from build123d import *

# Parameters (mm, degrees)
SKETCH1_R               = 101.6
BOSS_EXTRUDE1_DEPTH     = 76.2
FILLET1_R               = 12.7
CUT_EXTRUDE1_DEPTH      = 163.639355693
CUT_EXTRUDE1_DEPTH_BACK = 163.639355693
CUT_EXTRUDE2_DEPTH      = 163.63935574
CUT_EXTRUDE2_DEPTH_BACK = 163.63935574
SKETCH5_R               = 12.7


with BuildPart() as part:
    # Sketch1 → Boss-Extrude1 (new body)
    with BuildSketch(Plane.YZ):
        with Locations(Location((0, 0, 0), (0, 0, 90))):
            Circle(SKETCH1_R)
    extrude(amount=BOSS_EXTRUDE1_DEPTH)

    # Fillet1
    fillet1_edges = [part.edges().sort_by_distance(p)[0] for p in [
        (0, 0, -101.6),
        (76.2, 0, -101.6),
    ]]
    fillet(fillet1_edges, radius=FILLET1_R)

    # Sketch2 → Cut-Extrude1 (cut, two sides: drawn at the far end of the back side and taken through both)
    with BuildSketch(Plane.YZ.offset(76.2).offset(-CUT_EXTRUDE1_DEPTH_BACK)):
        with BuildLine():
            ThreePointArc((-24.232427185, 7.612455104), (-25.4, 0), (-24.232427185, -7.612455104))
            add(Edge.make_bspline(
                [(-24.232427185, -7.612455104), (-44.761154303, -23.370868648), (-69.597655338, -31.025898399)],
                knots=[0, 0, 0, 1, 1, 1], degree=2))
            ThreePointArc((-69.597655338, -31.025898399), (-76.2, 0), (-69.597655338, 31.025898399))
            add(Edge.make_bspline(
                [(-24.232427185, 7.612455104), (-44.761154303, 23.370868648), (-69.597655338, 31.025898399)],
                knots=[0, 0, 0, 1, 1, 1], degree=2))
        make_face()
        with BuildLine():
            ThreePointArc((18.708793098, 17.179669986), (12.7, 21.997045256), (5.523634087, 24.79212509))
            add(Edge.make_bspline(
                [(5.523634087, 24.79212509), (2.140811193, 50.449731053), (7.92961148, 75.786286766)],
                knots=[0, 0, 0, 1, 1, 1], degree=2))
            ThreePointArc((7.92961148, 75.786286766), (38.1, 65.991135768), (61.668043858, 44.760388367))
            add(Edge.make_bspline(
                [(18.708793098, 17.179669986), (42.620343109, 27.078862405), (61.668043858, 44.760388367)],
                knots=[0, 0, 0, 1, 1, 1], degree=2))
        make_face()
        with BuildLine():
            ThreePointArc((24.232427185, -7.612455104), (25.4, 0), (24.232427185, 7.612455104))
            add(Edge.make_bspline(
                [(24.232427185, 7.612455104), (44.761154303, 23.370868648), (69.597655338, 31.025898399)],
                knots=[0, 0, 0, 1, 1, 1], degree=2))
            ThreePointArc((69.597655338, 31.025898399), (76.2, 0), (69.597655338, -31.025898399))
            add(Edge.make_bspline(
                [(24.232427185, -7.612455104), (44.761154303, -23.370868648), (69.597655338, -31.025898399)],
                knots=[0, 0, 0, 1, 1, 1], degree=2))
        make_face()
        with BuildLine():
            ThreePointArc((-61.668043858, -44.760388367), (-38.1, -65.991135768), (-7.92961148, -75.786286766))
            add(Edge.make_bspline(
                [(-5.523634087, -24.79212509), (-2.140811193, -50.449731053), (-7.92961148, -75.786286766)],
                knots=[0, 0, 0, 1, 1, 1], degree=2))
            ThreePointArc((-5.523634087, -24.79212509), (-12.7, -21.997045256), (-18.708793098, -17.179669986))
            add(Edge.make_bspline(
                [(-18.708793098, -17.179669986), (-42.620343109, -27.078862405), (-61.668043858, -44.760388367)],
                knots=[0, 0, 0, 1, 1, 1], degree=2))
        make_face()
        with BuildLine():
            ThreePointArc((5.523634087, -24.79212509), (12.7, -21.997045256), (18.708793098, -17.179669986))
            add(Edge.make_bspline(
                [(18.708793098, -17.179669986), (42.620343109, -27.078862405), (61.668043858, -44.760388367)],
                knots=[0, 0, 0, 1, 1, 1], degree=2))
            ThreePointArc((61.668043858, -44.760388367), (38.1, -65.991135768), (7.92961148, -75.786286766))
            add(Edge.make_bspline(
                [(5.523634087, -24.79212509), (2.140811193, -50.449731053), (7.92961148, -75.786286766)],
                knots=[0, 0, 0, 1, 1, 1], degree=2))
        make_face()
        with BuildLine():
            ThreePointArc((-7.92961148, 75.786286766), (-38.1, 65.991135768), (-61.668043858, 44.760388367))
            add(Edge.make_bspline(
                [(-18.708793098, 17.179669986), (-42.620343109, 27.078862405), (-61.668043858, 44.760388367)],
                knots=[0, 0, 0, 1, 1, 1], degree=2))
            ThreePointArc((-18.708793098, 17.179669986), (-12.7, 21.997045256), (-5.523634087, 24.79212509))
            add(Edge.make_bspline(
                [(-5.523634087, 24.79212509), (-2.140811193, 50.449731053), (-7.92961148, 75.786286766)],
                knots=[0, 0, 0, 1, 1, 1], degree=2))
        make_face()
    extrude(amount=CUT_EXTRUDE1_DEPTH + CUT_EXTRUDE1_DEPTH_BACK, mode=Mode.SUBTRACT)

    # Sketch5 → Cut-Extrude2 (cut, two sides: drawn at the far end of the back side and taken through both)
    with BuildSketch(Plane.YZ.offset(76.2).offset(-CUT_EXTRUDE2_DEPTH_BACK)):
        with Locations(Location((0, 0, 0), (0, 0, 270))):
            Circle(SKETCH5_R)
    extrude(amount=CUT_EXTRUDE2_DEPTH + CUT_EXTRUDE2_DEPTH_BACK, mode=Mode.SUBTRACT)


solid = part.part
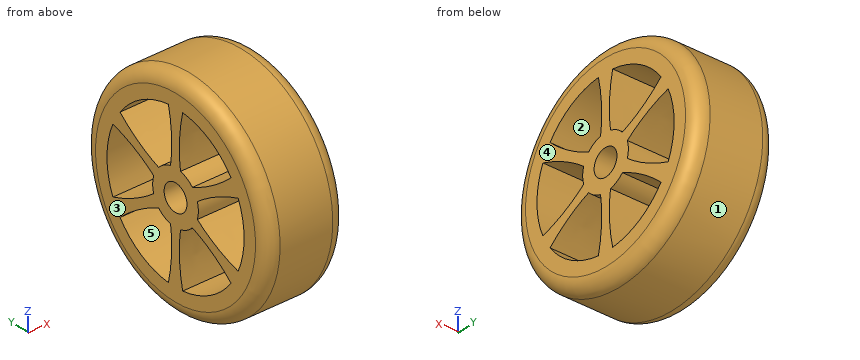
Check sheet for the modelled part. Datum: model origin and axes. Units: mm. Face numbers are marked on the shaded views. A direction names the side the tool comes from. Give positions to 0.01 mm unless a question says otherwise; leave off trailing zeros. Write each loop counter-clockwise with the first axis right and the second up, starting at its lowest first coordinate (ties: lowest second). Pieces come first, ordered by that corner, then holes. Notation, with made-up numbers: (-33.75, 21) -> (3.25, 21) arc R29 ccw to (3.25, 53) -> close; hole circle Ø4 at (27, 50.5). An arc over 180 degrees is marked (long way). Use one line per item in the form item = value. Start each with the question number.
1. Section check A-A (y = 0). Record the cut outline in (x, z), and give its area (3 significant figures).
2. Thickness scan on line 1 along Z through (x, y) = (47.5, 22); line 2 along Y through (x, z) = (30, -11.5); line 3 along Z through (x, y) = (30.5, -31). Record the ranges inside material, lowest first. Write a range as from..to.
3. Access from +Z, -Z, +X, -X, +Y, -Y to the whole of each face (thin tool, end or side, straight path). Record for the marked faces 4 and 5.
4. Go/stop test with flat-tipped pins: P1, Ø10, axis at x = 53, y = 61.5, coming from the +Z side; P2, Ø1.5, axis at x = 9.5, z = -55, coming from the +Y side; P3, Ø1.5, axis at x = 49, y = 42, coming from the +Z side; P4, Ø8, axis at y = 69, z = -24, coming from the +X side. Record where each tip stops, or that it passes through.
5. Section check B-B (z = 0). Record the cut outline in (x, y), and give its area (3 significant figures).
6. Section check C-C (x = 49). Count the separate pieces of the cut face and the enclosed holes in it, and give its area (3 significant figures).
7. Mould release check, pull along Z, two halves, no side actions. Record for the marked faces 1, 2 and 3: pulls with the +Z half, pulls with the -Z half, needs draft (parallel to the pull), parting line crosses it, or undercut.
Conclusion:
q1.outline = (0, -88.9) arc R12.7 ccw to (12.7, -101.6) -> (63.5, -101.6) arc R12.7 ccw to (76.2, -88.9) -> (76.2, -12.7) -> (0, -12.7) -> close; (0, 12.7) -> (76.2, 12.7) -> (76.2, 88.9) arc R12.7 ccw to (63.5, 101.6) -> (12.7, 101.6) arc R12.7 ccw to (0, 88.9) -> close
q1.area = 13,400 mm²
q2.line_1 = -99.19..-72.96, -18.59..18.59, 72.96..99.19
q2.line_2 = -100.95..-75.33, -29.54..-5.39, 5.39..29.54, 75.33..100.95
q2.line_3 = -96.76..-69.61, -22.95..-12.51, 12.51..22.95, 69.61..96.76
q3.face_4 = +Z, -Z, +X, +Y, -Y
q3.face_5 = +X, -X
q4.P1 = 84.44
q4.P2 = 85.47
q4.P3 = 92.85
q4.P4 = 76.2
q5.outline = (0, -88.9) arc R12.7 ccw to (12.7, -101.6) -> (63.5, -101.6) arc R12.7 ccw to (76.2, -88.9) -> (76.2, -76.2) -> (0, -76.2) -> close; (0, -25.4) -> (76.2, -25.4) -> (76.2, -12.7) -> (0, -12.7) -> close; (0, 12.7) -> (76.2, 12.7) -> (76.2, 25.4) -> (0, 25.4) -> close; (0, 76.2) -> (76.2, 76.2) -> (76.2, 88.9) arc R12.7 ccw to (63.5, 101.6) -> (12.7, 101.6) arc R12.7 ccw to (0, 88.9) -> close
q5.area = 5,670 mm²
q6.separate_pieces = 1
q6.enclosed_holes = 7
q6.area = 18,900 mm²
q7.face_1 = parting line crosses it
q7.face_2 = undercut
q7.face_3 = needs draft
